Geometry check sheet. Reference: the model listing, model coordinates, mm. Face numbers are marked on the shaded views. A direction names the side the tool comes from. Round coordinates to 2 decimals unless told otherwise and drop trailing zeros. Write each loop counter-clockwise with the first axis right and the second up, starting at its lowest first coordinate (ties: lowest second). Pieces come first, ordered by that corner, then holes.
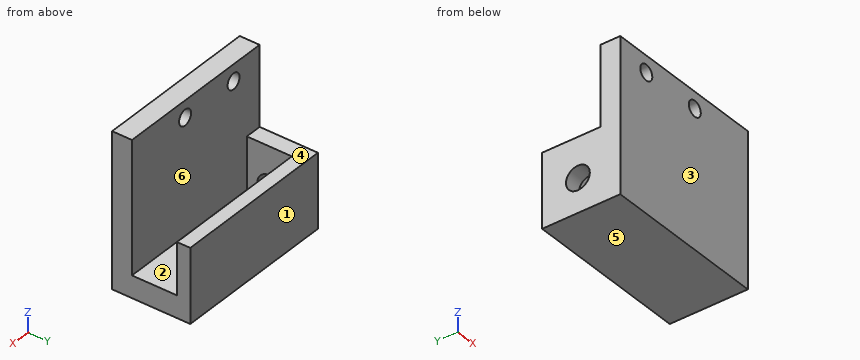
from build123d import *

# Parameters (mm, degrees)
SKETCH1_W           = 25
SKETCH1_H           = 20
SKETCH1_R           = 1.175
BOSS_EXTRUDE2_DEPTH = 3
SKETCH3_W           = 2.5
SKETCH3_H           = 8
BOSS_EXTRUDE3_DEPTH = 6.8
SKETCH5_W           = 2.5
SKETCH5_H           = 6.8
BOSS_EXTRUDE5_DEPTH = 6.8
SKETCH7_R           = 1.8
CUT_EXTRUDE1_DEPTH  = 6.8
SKETCH8_W           = 7
SKETCH8_H           = 6.8
BOSS_EXTRUDE6_DEPTH = 22.5
SKETCH9_W           = 25
SKETCH9_H           = 14.8
BOSS_EXTRUDE7_DEPTH = 2
SKETCH10_W          = 3.676013555
SKETCH10_H          = 11.8
CUT_EXTRUDE2_DEPTH  = 36


with BuildPart() as part:
    # Sketch1 → Boss-Extrude2 (new body)
    with BuildSketch(Plane(origin=(0, 0, 0), x_dir=(1, 0, 0), z_dir=(0, 1, 0))):
        with Locations((12.5, 10)):
            Rectangle(SKETCH1_W, SKETCH1_H)
        with Locations(Location((5.1, 2.5, 0), (0, 0, 270))):
            Circle(SKETCH1_R, mode=Mode.SUBTRACT)
        with Locations(Location((14.6, 2.5, 0), (0, 0, 270))):
            Circle(SKETCH1_R, mode=Mode.SUBTRACT)
    extrude(amount=BOSS_EXTRUDE2_DEPTH)

    # Sketch3 → Boss-Extrude3 (add)
    with BuildSketch(Plane(origin=(0, 3, 0), x_dir=(1, 0, 0), z_dir=(0, 1, 0))):
        with Locations((1.25, 16)):
            Rectangle(SKETCH3_W, SKETCH3_H)
    extrude(amount=BOSS_EXTRUDE3_DEPTH)

    # Sketch5 → Boss-Extrude5 (add)
    with BuildSketch(Plane(origin=(0, 0, -20), x_dir=(-1, 0, 0), z_dir=(0, 0, -1))):
        Polygon((0, 0), (0, 3), (-2.5, 3), (-25, 3), (-25, 0), align=None)
        with Locations((-1.25, 6.4)):
            Rectangle(SKETCH5_W, SKETCH5_H)
    extrude(amount=BOSS_EXTRUDE5_DEPTH)

    # Sketch7 → Cut-Extrude1 (cut)
    with BuildSketch(Plane.ZY):
        with Locations((-18, 6.4)):
            Circle(SKETCH7_R)
    extrude(amount=-CUT_EXTRUDE1_DEPTH, mode=Mode.SUBTRACT)

    # Sketch8 → Boss-Extrude6 (add)
    with BuildSketch(Plane(origin=(2.5, 0, 0), x_dir=(0, 0, -1), z_dir=(1, 0, 0))):
        with Locations((23.3, 6.4)):
            Rectangle(SKETCH8_W, SKETCH8_H)
    extrude(amount=BOSS_EXTRUDE6_DEPTH)

    # Sketch9 → Boss-Extrude7 (add)
    with BuildSketch(Plane(origin=(0, 9.8, 0), x_dir=(1, 0, 0), z_dir=(0, 1, 0))):
        with Locations((12.5, 19.4)):
            Rectangle(SKETCH9_W, SKETCH9_H)
    extrude(amount=BOSS_EXTRUDE7_DEPTH)

    # Sketch10 → Cut-Extrude2 (cut)
    with BuildSketch(Plane(origin=(25, 0, 0), x_dir=(0, 0, -1), z_dir=(1, 0, 0))):
        with Locations((24.961993222, 5.9)):
            Rectangle(SKETCH10_W, SKETCH10_H)
    extrude(amount=-CUT_EXTRUDE2_DEPTH, mode=Mode.SUBTRACT)


solid = part.part
1. Release check for a two-part mould opening along Y. For the marked faces 1, 2 and 3 record: +Y half, -Y half, draft (parallel to the pull), parting line (faces both ways), or undercut.
2. Section check B-B (z = -2.5). Record the cut outline in (x, y) (3 decimals), plus the area to 3 significant figures.
3. Scan lines: line 1 along X through (y, z) = (1.8, -2.5) (3 decimals); line 2 along Y through (x, z) = (8.5, -15); line 3 along Y through (x, z) = (1.8, -18). Record each from-to range of solid material in increasing order.
4. Access from +Z, -Z, +X, -X, +Y, -Y to the whole of each face (thin tool, end or side, straight path). Record for the marked faces 4, 5 and 6.
5. Depth check by flat-ended pin: pin 1 Ø3 at (y, z) = (6.4, -18) entering from +X; pin 2 Ø2 at (x, y) = (9.5, 7) entering from +Z. Enter the tip coordinate at first touch or a pass-through.
6. Section check C-C (x = 5.1). Record the cut outline in (y, z) (3 decimals).
7. Section check D-D (y = 3.5). Record the cut outline in (x, z), plus the area to 3 significant figures.
8. Section check A-A (z = -18). Record the cut outline in (x, y), plus the area to 3 significant figures.
Results below:
1. face 1: +Y half
1. face 2: undercut
1. face 3: -Y half
2. outline: (0, 0) - (3.925, 0) - (3.925, 3) - (0, 3) - close; (6.275, 0) - (13.425, 0) - (13.425, 3) - (6.275, 3) - close; (15.775, 0) - (25, 0) - (25, 3) - (15.775, 3) - close
2. area: 60.9 mm2
3. line 1: x = 0 to 3.925, 6.275 to 13.425, 15.775 to 25
3. line 2: y = 0 to 3, 9.8 to 11.8
3. line 3: y = 0 to 4.6, 8.2 to 11.8
4. face 4: +Z, +X, -X, +Y
4. face 5: -Z, +X, -X, +Y, -Y
4. face 6: +Z, +X
5. pin 1: passes through
5. pin 2: stops at z = -19.8
6. outline: (0, -23.124) - (11.8, -23.124) - (11.8, -12) - (9.8, -12) - (9.8, -19.8) - (3, -19.8) - (3, -3.675) - (0, -3.675) - close; (0, -1.325) - (3, -1.325) - (3, 0) - (0, 0) - close
7. outline: (0, -23.12) - (25, -23.12) - (25, -19.8) - (2.5, -19.8) - (2.5, -12) - (0, -12) - close
7. area: 103 mm2
8. outline: (0, 0) - (25, 0) - (25, 3) - (2.5, 3) - (2.5, 4.6) - (0, 4.6) - close; (0, 8.2) - (2.5, 8.2) - (2.5, 9.8) - (25, 9.8) - (25, 11.8) - (0, 11.8) - close
8. area: 133 mm2
